Can you work these out from the drawing? Everything is in mm from the part's minimum corner. A direction names the side the tool comes from. Round coordinates to 2 decimals unless told otherwise and drop trailing zeros. Loops run counter-clockwise (first coordinate to the right, second up) from the corner with the lowest first, then second, coordinate; pieces in that order, holes last. Notation, with made-up numbers: (7.25, -29.75) - (18.25, -29.75) arc R19 ccw to (18.25, -13.75) - close; hole circle Ø8 at (28.5, 37). An arc over 180 degrees is marked (long way). Answer as a JSON object with one key per item and string values. Group by question number.
1) I want a section at D-D, the plane z = 17. Please give me the cut outline in (x, y), then the cut area to 3 significant figures.
2) I want a section at C-C, the plane y = 32. Please give me the cut outline in (x, z).
3) If I drill on line 1 along Y through (x, z) = (10.5, 51); line 2 along Z through (x, y) = (12.5, 38); line 3 along X through (y, z) = (13, 39), over which ranges is the centre line in solid material (lowest first)? Write a range as [from, to].
4) I want a section at A-A, the plane x = 20.5. Please give me the cut outline in (y, z), then the cut area to 3 significant figures.
5) Which directions (+Z, -Z, +X, -X, +Y, -Y) give clear straight access to the entire face, cutting with the end or side of a thin tool? Please do the marked faces 1, 2, 3, 4 and 5.
6) Will these pins go through, and if not, where does the flat tip stop? P1, Ø3, axis at x = 3, y = 9, coming from the -Z side; P2, Ø1, axis at x = 16.5, y = 31.5, coming from the +Z side; P3, Ø1.8, axis at x = 2, y = 10.5, coming from the +Z side.
7) I want a section at B-B, the plane z = 25. Please give me the cut outline in (x, y).
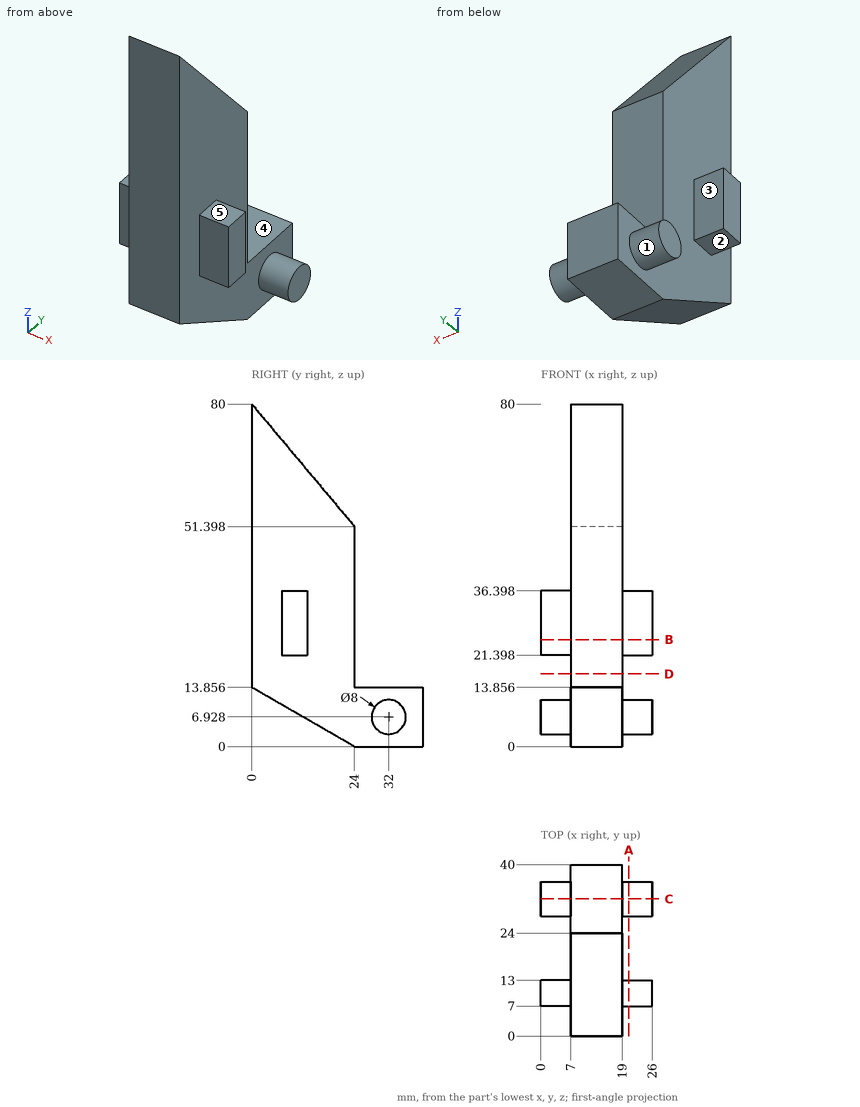
Outcome:
{
 "1": {"outline": "(7, 0) - (19, 0) - (19, 24) - (7, 24) - close", "area": "288 mm^2"},
 "2": {"outline": "(0, 2.93) - (7, 2.93) - (7, 0) - (19, 0) - (19, 2.93) - (26, 2.93) - (26, 10.93) - (19, 10.93) - (19, 13.86) - (7, 13.86) - (7, 10.93) - (0, 10.93) - close"},
 "3": {"line 1": "[0, 24]", "line 2": "[0, 13.86]", "line 3": "[7, 19]"},
 "4": {"outline": "(7, 21.4) - (13, 21.4) - (13, 36.4) - (7, 36.4) - close; circle Ø8 at (32, 6.93)", "area": "140 mm^2"},
 "5": {"face 1": "-X", "face 2": "-Z, -X, +Y, -Y", "face 3": "+Z, -Z, -X, +Y", "face 4": "+Z, +X, -X, +Y", "face 5": "+Z, +X, +Y, -Y"},
 "6": {"P1": "z = 21.4", "P2": "z = 13.86", "P3": "z = 36.4"},
 "7": {"outline": "(0, 7) - (7, 7) - (7, 0) - (19, 0) - (19, 7) - (26, 7) - (26, 13) - (19, 13) - (19, 24) - (7, 24) - (7, 13) - (0, 13) - close"}
}
